Geometry check sheet. Reference: the model listing, model coordinates, mm. A direction names the side the tool comes from. Give positions to 0.01 mm unless a question says otherwise; leave off trailing zeros. Order: outer loops, then holes, each group sorted by start corner. A loop starts at its lowest first (then second) coordinate and runs counter-clockwise, first axis right, second up.
```python
from build123d import *

# Parameters (mm, degrees)
BASEHEAD_DEPTH   = 14
HEADFILLET_R     = 0.8
BASEBODYFILLET_R = 0.8


with BuildPart() as part:
    # HexSke → BaseHead (new body)
    with BuildSketch(Plane(origin=(0, 0, 0), x_dir=(0, 0, -1), z_dir=(1, 0, 0))):
        Polygon((12, 6.92820323), (12, -6.92820323), (0, -13.856406461), (-12, -6.92820323), (-12, 6.92820323), (0, 13.856406461), align=None)
    extrude(amount=BASEHEAD_DEPTH)

    # BodySke → BaseBody (revolve)
    with BuildSketch(Plane.XY, mode=Mode.PRIVATE) as basebody_sk:
        Polygon((0, 0), (94, 0), (94, 7.5), (83.64, 7.5), (81.14, 10), (0, 10), align=None)
    revolve(basebody_sk.sketch.rotate(Axis((0, 0, 0), (1, 0, 0)), 90), axis=Axis((0, 0, 0), (1, 0, 0)))

    # HeadChamSke → HeadChamfer (revolve, cut)
    with BuildSketch(Plane.XY):
        Polygon((0, 12), (3.958548116, 18.856406461), (3.958548116, 23.856406461), (-10, 23.856406461), (-10, 12), align=None)
    revolve(axis=Axis((0, 0, 0), (1, 0, 0)), mode=Mode.SUBTRACT)

    # HeadFillet
    headfillet_edges = [part.edges().sort_by_distance(p)[0] for p in [
        (14, 0, -10),
    ]]
    fillet(headfillet_edges, radius=HEADFILLET_R)

    # BaseBodyFillet
    basebodyfillet_edges = [part.edges().sort_by_distance(p)[0] for p in [
        (94, 0, -7.5),
    ]]
    fillet(basebodyfillet_edges, radius=BASEBODYFILLET_R)


solid = part.part
```
Q1. Gauge pin test, flat ends, axial feed: P1, Ø1.5, axis at x = 82.5, y = 7.5, coming from the -Z side; P2, Ø4, axis at x = 53.5, y = 0, coming from the -Z side; P3, Ø2, axis at x = 77.5, y = 6, coming from the +Z side. Record the tip position at first contact, or that the pin passes through.
Q2. Thickness scan on L1, parallel to Y at x = 62, z = -0.5; L2, parallel to Y at x = 43.5, z = -8; L3, parallel to X at y = -6, z = 8.5. Record the ranges inside material, lowest first.
Q3. Cross-section at B-B, the plane x = 84.5. Record the boundary of the cut face in (y, z).
Q4. Cross-section at C-C, the plane x = 42.5. Record the boundary of the cut face in (y, z), and give its area (3 significant figures).
Q5. Access from +Z, -Z, +X, -X, +Y, -Y to the whole of each face (thin tool, end or side, straight path). Record for faces 1 (the face through (0.26, -6.2, 10.8)), 2 (the face through (88.353, -6.324, 4.032)).
Q6. Cross-section at A-A, the plane x = 9.5. Record the boundary of the cut face in (y, z), and give its area (3 significant figures).
Answers follow:
1. P1: stops at z = -5.97
1. P2: stops at z = -10
1. P3: stops at z = 8.66
2. L1: y = -9.99 to 9.99
2. L2: y = -6 to 6
2. L3: x = 0 to 14.1
3. outline: circle Ø15 at (0, 0)
4. outline: circle Ø20 at (0, 0)
4. area: 314 mm2
5. face 1: +Z, -X, -Y
5. face 2: +X
6. outline: (-13.86, 0) - (-6.93, -12) - (6.93, -12) - (13.86, 0) - (6.93, 12) - (-6.93, 12) - close
6. area: 499 mm2
